Build history of the part. All positions in model axes, mm. A direction names the side the tool comes from. Round coordinates to 2 decimals unless told otherwise and drop trailing zeros. Loops run counter-clockwise (first coordinate to the right, second up) from the corner with the lowest first, then second, coordinate; pieces in that order, holes last.
from build123d import *

# Parameters (mm, degrees)
SKETCH1_R           = 56
BOSS_EXTRUDE1_DEPTH = 10
SKETCH2_R           = 10
BOSS_EXTRUDE2_DEPTH = 30
SKETCH3_R           = 5
CUT_EXTRUDE1_DEPTH  = 10


with BuildPart() as part:
    # Sketch1 → Boss-Extrude1 (new body)
    with BuildSketch(Plane.XY):
        Circle(SKETCH1_R)
    extrude(amount=BOSS_EXTRUDE1_DEPTH)

    # Sketch2 → Boss-Extrude2 (add)
    with BuildSketch(Plane.XY.offset(10)):
        Circle(SKETCH2_R)
    extrude(amount=BOSS_EXTRUDE2_DEPTH)

    # Sketch3 → Cut-Extrude1 (cut)
    with BuildSketch(Plane.XY.offset(10)):
        with Locations((36, 0)):
            Circle(SKETCH3_R)
        with Locations((-18, 31.176914536)):
            Circle(SKETCH3_R)
        with Locations((-18, -31.176914536)):
            Circle(SKETCH3_R)
    extrude(amount=-CUT_EXTRUDE1_DEPTH, mode=Mode.SUBTRACT)


solid = part.part
(1) Slice it at A-A on y = 0. List the corners of the cut face in (x, z).
Responses:
outline: (-56, 0) - (31, 0) - (31, 10) - (10, 10) - (10, 40) - (-10, 40) - (-10, 10) - (-56, 10) - close; (41, 0) - (56, 0) - (56, 10) - (41, 10) - close
(2) Slice it at D-D on x = 0. List the corners of the cut face in (y, z), plus the area to 3 significant figures.
Responses:
outline: (-56, 0) - (56, 0) - (56, 10) - (10, 10) - (10, 40) - (-10, 40) - (-10, 10) - (-56, 10) - close
area: 1,720 mm2
(3) Probe line 1 (Y direction, x = -18, z = 5); line 2 (Z direction, x = 14.5, y = 33); line 3 (Y direction, x = 36, z = 7). List the from-to ranges inside material, lowest first.
Responses:
line 1: y = -53.03 to -36.18, -26.18 to 26.18, 36.18 to 53.03
line 2: z = 0 to 10
line 3: y = -42.9 to -5, 5 to 42.9
(4) Slice it at C-C on x = -18. List the corners of the cut face in (y, z), plus the area to 3 significant figures.
Responses:
outline: (-53.03, 0) - (-36.18, 0) - (-36.18, 10) - (-53.03, 10) - close; (-26.18, 0) - (26.18, 0) - (26.18, 10) - (-26.18, 10) - close; (36.18, 0) - (53.03, 0) - (53.03, 10) - (36.18, 10) - close
area: 861 mm2
(5) Pull direction X, two halves, no side cores. Call faces 1 (the face through (-19.1, 26.3, 5.1)), 2 (the face through (-1, 1, 0)), 3 (the face through (51.73, -21.45, 4.93)): +X half, -X half, draft (parallel to the pull), parting line (faces both ways), or undercut.
Responses:
face 1: undercut
face 2: draft
face 3: parting line
(6) Pin check, flat tips, straight feed: P1, Ø5, axis at y = 25, z = 10, coming from the +X side; P2, Ø4, axis at y = 7.5, z = 11, coming from the +X side; P3, Ø16, axis at x = -18, y = 31.18, coming from the +Z side; P4, Ø8, axis at x = 36, y = 0, coming from the +Z side. Stop position of each tip, or through.
Responses:
P1: stops at x = 51.28
P2: stops at x = 55.7
P3: stops at z = 10
P4: passes through
(7) Slice it at B-B on x = 34. List the corners of the cut face in (y, z).
Responses:
outline: (-44.5, 0) - (-4.58, 0) - (-4.58, 10) - (-44.5, 10) - close; (4.58, 0) - (44.5, 0) - (44.5, 10) - (4.58, 10) - close
(8) Which spindle directions (+Z, -Z, +X, -X, +Y, -Y) get a long thin tool onto all of the face, cutting with end or side? Do faces 4 (the face through (-19.08, -36.06, 5.07)), 5 (the face through (-2.17, -9.76, 24.79)). Say none if no direction does.
Responses:
face 4: +Z, -Z
face 5: +Z
